For this review, take the finished solid that the model builds, in its own axes (mm). A direction names the side the tool comes from. Round coordinates to 2 decimals unless told otherwise and drop trailing zeros. Write each loop counter-clockwise with the first axis right and the second up, starting at its lowest first coordinate (ties: lowest second). Pieces come first, ordered by that corner, then holes. Notation, with made-up numbers: M -13,5.25 L 12,5.25 A5 cw 12,9.25 Z; hole C 35.5,-18.75 d2. An arc over 180 degrees is marked long. One line per question, with ' | ' between items.
```python
from build123d import *

# Parameters (mm, degrees)
SKETCH2_W               = 184
SKETCH2_H               = 332.5
BOSS_EXTRUDE1_DEPTH     = 5
SKETCH3_W               = 36.5
SKETCH3_H               = 5
SKETCH3_W_2             = 62.5
CUT_EXTRUDE1_DEPTH      = 5
CUT_EXTRUDE2_DEPTH      = 10
SKETCH5_R               = 2.1
CUT_EXTRUDE3_DEPTH      = 10
ENL_V_MAT_EXTRU_2_DEPTH = 10


with BuildPart() as part:
    # Sketch2 → Boss-Extrude1 (new body)
    with BuildSketch(Plane.XY):
        Rectangle(SKETCH2_W, SKETCH2_H)
    extrude(amount=BOSS_EXTRUDE1_DEPTH)

    # Sketch3 → Cut-Extrude1 (cut)
    with BuildSketch(Plane.XY.offset(5)):
        with Locations((-73.75, 163.75)):
            Rectangle(SKETCH3_W, SKETCH3_H)
        with Locations((60.75, 163.75)):
            Rectangle(SKETCH3_W_2, SKETCH3_H)
        with Locations((60.75, 98.75)):
            Rectangle(SKETCH3_W_2, SKETCH3_H)
        with BuildLine():
            Line((27.5, -141.25), (27.5, -166.25))
            Line((27.5, -166.25), (-53.5, -166.25))
            Line((-53.5, -166.25), (-53.5, -141.25))
            ThreePointArc((-53.5, -141.25), (-13, -100.75), (27.5, -141.25))
        make_face()
        with Locations((-73.75, 98.75)):
            Rectangle(SKETCH3_W, SKETCH3_H)
    extrude(amount=-CUT_EXTRUDE1_DEPTH, mode=Mode.SUBTRACT)

    # Sketch4 → Cut-Extrude2 (cut)
    with BuildSketch(Plane.XY.offset(5)):
        Polygon((55.75, 161.25), (55.75, 151.25), (58.65, 151.25), (58.65, 146.25), (62.85, 146.25), (62.85, 151.25), (65.75, 151.25), (65.75, 161.25), align=None)
        Polygon((-78.75, 161.25), (-78.75, 151.25), (-75.85, 151.25), (-75.85, 146.25), (-71.65, 146.25), (-71.65, 151.25), (-68.75, 151.25), (-68.75, 161.25), align=None)
        Polygon((65.75, -166.25), (65.75, -156.25), (62.85, -156.25), (62.85, -151.25), (58.65, -151.25), (58.65, -156.25), (55.75, -156.25), (55.75, -166.25), align=None)
        Polygon((-68.75, -166.25), (-68.75, -156.25), (-71.65, -156.25), (-71.65, -151.25), (-75.85, -151.25), (-75.85, -156.25), (-78.75, -156.25), (-78.75, -166.25), align=None)
    extrude(amount=-CUT_EXTRUDE2_DEPTH, mode=Mode.SUBTRACT)

    # Sketch5 → Cut-Extrude3 (cut)
    with BuildSketch(Plane.XY.offset(5)):
        with Locations((-13, 98.75)):
            Circle(SKETCH5_R)
    extrude(amount=-CUT_EXTRUDE3_DEPTH, mode=Mode.SUBTRACT)

    # Esquisse2 → Enlèv. mat.-Extru.2 (cut)
    with BuildSketch(Plane.XY.offset(5)):
        with BuildLine():
            Line((10.470660362, -8.273773364), (10.470660362, -59.567669296))
            ThreePointArc((10.470660362, -59.567669296), (51.484945295, -58.532619163), (92, -64.995841242))
            Line((92, -64.995841242), (92, -3.75037767))
            ThreePointArc((92, -3.75037767), (50.880784547, 0.378228003), (10.470660362, -8.273773364))
        make_face()
    extrude(amount=-ENL_V_MAT_EXTRU_2_DEPTH, mode=Mode.SUBTRACT)


solid = part.part
```
Item 1: Take a section at B-B (y = -38). Write out the cut boundary in (x, z).
Results:
outline: M -92,0 L 10.47,0 L 10.47,5 L -92,5 Z
Item 2: Machinability: for faces 4 (the face through (50.911, -58.495, 2.535)), 5 (the face through (-1, 2, 0)), which of the approach directions +Z, -Z, +X, -X, +Y, -Y give a long, thin tool a straight path to every point of the face, cutting with its end or side? Answer none if there is none.
Results:
face 4: +Z, -Z | face 5: -Z, +X, -X, +Y, -Y
Item 3: To check wall thickness, follow line 1 along Y through (x, z) = (-13, 3.65); line 2 along Y through (x, z) = (40, 2.15); line 3 along X through (y, z) = (-46, 3.7). State the ranges of each line that lie inside material, in increasing order. Write a range as from..to.
Results:
line 1: -100.75..96.65, 100.85..166.25 | line 2: -166.25..-58.06, -0.67..96.25, 101.25..161.25 | line 3: -92..10.47
Item 4: Take a section at A-A (y = -138). Write out the cut boundary in (x, z), then the cut area to 3 significant figures.
Results:
outline: M -92,0 L -53.37,0 L -53.37,5 L -92,5 Z; M 27.37,0 L 92,0 L 92,5 L 27.37,5 Z | area: 516 mm2
Item 5: Take a section at C-C (x = 4). Write out the cut boundary in (y, z).
Results:
outline: M -104.49,0 L 166.25,0 L 166.25,5 L -104.49,5 Z
Item 6: Mouldability with a two-part tool opening along Y and no side actions: class faces 1 (the face through (51.46, 0.41, 2.54)), 2 (the face through (-1, 2, 5)), 3 (the face through (-13.89, -100.76, 2.54)) as +Y half, -Y half, draft (parallel to the pull), parting line (faces both ways), or undercut.
Results:
face 1: undercut | face 2: draft | face 3: -Y half
Item 7: Insertion check: pin 1 Ø1.5 at (x, z) = (72.5, 1.5) entering from +Y; pin 2 Ø1.4 at (x, z) = (57, 2.5) entering from -Y; pin 3 Ø1.5 at (x, z) = (-75.5, 1.5) entering from +Y. Each pin has a flat end and moves straight along its axis. Give the tip position at first contact, or say it passes through.
Results:
pin 1: y = 161.25 | pin 2: y = -156.25 | pin 3: y = 151.25
